Geometry: final body of the model. Coordinates: model frame, mm. Face numbers are marked on the shaded views. A direction names the side the tool comes from. Round coordinates to 2 decimals unless told otherwise and drop trailing zeros. Loops run counter-clockwise (first coordinate to the right, second up) from the corner with the lowest first, then second, coordinate; pieces in that order, holes last. Notation, with made-up numbers: (-30, 31.5) -> (-20, 31.5) arc R7 ccw to (-20, 39.5) -> close; hole circle Ø7 at (74.5, -19.75). An arc over 180 degrees is marked (long way). Answer in a Markdown table with one row per item.
```python
from build123d import *

# Parameters (mm, degrees)
ESQUISSE1_R             = 10
BOSS_EXTRU_1_DEPTH      = 8.2
ESQUISSE2_R             = 8.354
ENL_V_MAT_EXTRU_1_DEPTH = 5.65
ESQUISSE3_W             = 38.1
ESQUISSE3_H             = 38.1
BOSS_EXTRU_3_DEPTH      = 1.5
ESQUISSE4_R             = 2.5
ENL_V_MAT_EXTRU_2_DEPTH = 2


with BuildPart() as part:
    # Esquisse1 → Boss.-Extru.1 (new body)
    with BuildSketch(Plane(origin=(0, 0, 0), x_dir=(1, 0, 0), z_dir=(0, 1, 0))):
        Circle(ESQUISSE1_R)
    extrude(amount=-BOSS_EXTRU_1_DEPTH)

    # Esquisse2 → Enlèv. mat.-Extru.1 (cut)
    with BuildSketch(Plane(origin=(0, 0, 0), x_dir=(1, 0, 0), z_dir=(0, 1, 0))):
        Circle(ESQUISSE2_R)
    extrude(amount=-ENL_V_MAT_EXTRU_1_DEPTH, mode=Mode.SUBTRACT)

    # Esquisse3 → Boss.-Extru.3 (add)
    with BuildSketch(Plane(origin=(0, -8.2, 0), x_dir=(-1, 0, 0), z_dir=(0, -1, 0))):
        Rectangle(ESQUISSE3_W, ESQUISSE3_H)
    extrude(amount=-BOSS_EXTRU_3_DEPTH)

    # Esquisse4 → Enlèv. mat.-Extru.2 (cut)
    with BuildSketch(Plane(origin=(0, -6.7, 0), x_dir=(1, 0, 0), z_dir=(0, 1, 0))):
        with Locations((-11.55, 11.55)):
            Circle(ESQUISSE4_R)
        with Locations((11.55, 11.55)):
            Circle(ESQUISSE4_R)
        with Locations((11.55, -11.55)):
            Circle(ESQUISSE4_R)
        with Locations((-11.55, -11.55)):
            Circle(ESQUISSE4_R)
    extrude(amount=-ENL_V_MAT_EXTRU_2_DEPTH, mode=Mode.SUBTRACT)


solid = part.part
```
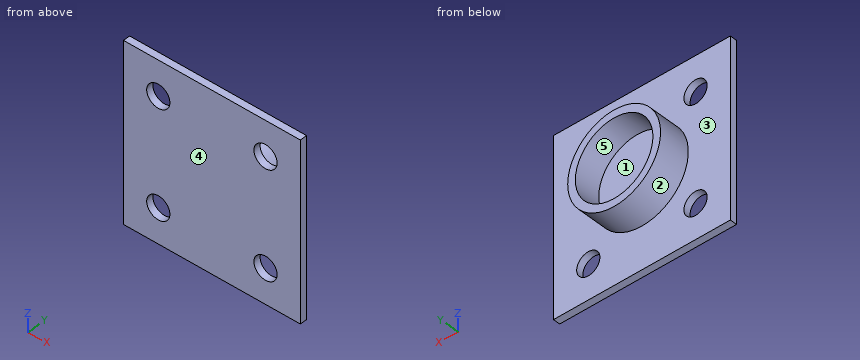
Item 1: Set-up query: the marked faces 4 and 5. Return all of +Z, -Z, +X, -X, +Y, -Y with unobstructed straight access to the full face (end or side cutting, diameter ignored); none if empty.
Ans:
| item | result |
|---|---|
| face 4 | +Z, -Z, +X, -X, -Y |
| face 5 | +Y |
Item 2: Section query C-C, the plane y = -5. Output: boundary loops of the cut face in (x, z).
Ans:
| item | result |
|---|---|
| outline | circle Ø20 at (0, 0); hole circle Ø16.71 at (0, 0) |
Item 3: Mould query, pull axis Z, two halves, no side actions, for the marked faces 1, 2 and 3. Classes: released by +Z, released by -Z, zero draft, split by the parting line, or undercut.
Ans:
| item | result |
|---|---|
| face 1 | undercut |
| face 2 | split by the parting line |
| face 3 | zero draft |
Item 4: Section query D-D, the plane x = 0. Output: boundary loops of the cut face in (y, z).
Ans:
| item | result |
|---|---|
| outline | (-8.2, -19.05) -> (-6.7, -19.05) -> (-6.7, -10) -> (0, -10) -> (0, -8.35) -> (-5.65, -8.35) -> (-5.65, 8.35) -> (0, 8.35) -> (0, 10) -> (-6.7, 10) -> (-6.7, 19.05) -> (-8.2, 19.05) -> close |
Item 5: Section query B-B, the plane z = -11.55. Output: boundary loops of the cut face in (x, y).
Ans:
| item | result |
|---|---|
| outline | (-19.05, -8.2) -> (-14.05, -8.2) -> (-14.05, -6.7) -> (-19.05, -6.7) -> close; (-9.05, -8.2) -> (9.05, -8.2) -> (9.05, -6.7) -> (-9.05, -6.7) -> close; (14.05, -8.2) -> (19.05, -8.2) -> (19.05, -6.7) -> (14.05, -6.7) -> close |
Item 6: Section query A-A, the plane x = -11.55. Output: boundary loops of the cut face in (y, z).
Ans:
| item | result |
|---|---|
| outline | (-8.2, -19.05) -> (-6.7, -19.05) -> (-6.7, -14.05) -> (-8.2, -14.05) -> close; (-8.2, -9.05) -> (-6.7, -9.05) -> (-6.7, 9.05) -> (-8.2, 9.05) -> close; (-8.2, 14.05) -> (-6.7, 14.05) -> (-6.7, 19.05) -> (-8.2, 19.05) -> close |
Item 7: First-contact query: P1, Ø2, axis at y = -1, z = 8.5, coming from the +X side; P2, Ø6, axis at x = 10, z = 10.5, coming from the +Y side; P3, Ø4, axis at x = 11.55, z = 11.55, coming from the -Y side; P4, Ø8.5, axis at x = 2.5, z = 1, coming from the +Y side. Flat tips, straight axial feed; report the tip coordinate or a pass-through.
Ans:
| item | result |
|---|---|
| P1 | x = 6.61 |
| P2 | y = -6.7 |
| P3 | through |
| P4 | y = -5.65 |
Item 8: Ray query, L1, parallel to Z at x = -11.55, y = -7.8; L2, parallel to X at y = -4.2, z = 0. Return the intervals inside material, ascending.
Ans:
| item | result |
|---|---|
| L1 | -19.05 to -14.05, -9.05 to 9.05, 14.05 to 19.05 |
| L2 | -10 to -8.35, 8.35 to 10 |
